Can you work these out from the drawing? Everything is in mm from the part's minimum corner. Give positions to 0.01 mm unless a question says otherwise; leave off trailing zeros. Loops run counter-clockwise (first coordinate to the right, second up) from the corner with the lowest first, then second, coordinate; pieces in that order, holes last.
Q1. If we section it at D-D (z = 20.5): Please give me the cut outline in (x, y), plus the area to 3 significant figures.
Q2. If we section it at A-A (y = 12): Please give me the cut outline in (x, z), plus the area to 4 significant figures.
Q3. Will this pin go through, and if not, where does the flat tip stop? P1, Ø1.5, axis at x = 1.5, z = 18, coming from the -Y side.
Q4. We'd pull the mould along Z, two halves only. Please class the marked faces 1, 2 and 3: +Z half, -Z half, draft (parallel to the pull), parting line (faces both ways), or undercut.
Q5. If we section it at C-C (x = 0.4): Please give me the cut outline in (y, z), plus the area to 3 significant figures.
Q6. I need wall thicknesses on line 1 (Y direction, x = 1.2, z = 12); line 2 (X direction, y = 13.5, z = 21.25). Which ranges of each line are inside material? Lowest first, please.
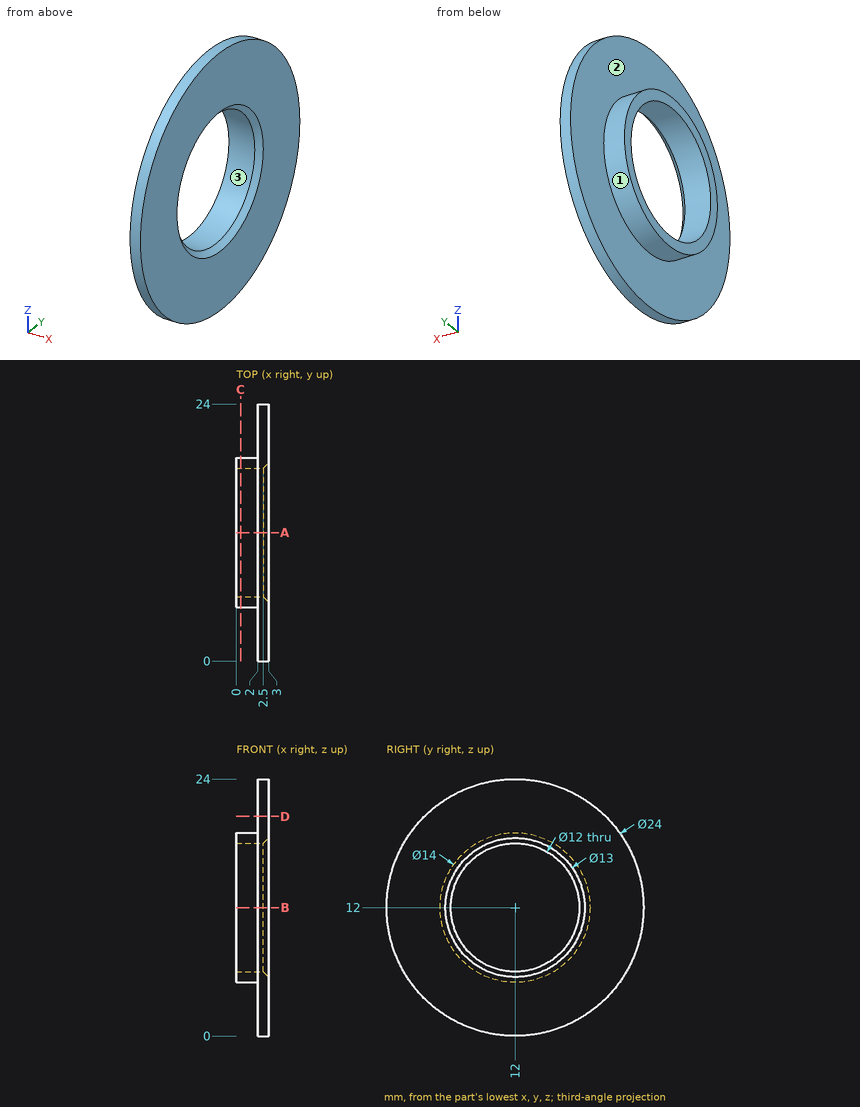
Check sheet entries:
1. outline: (2, 3.53) - (3, 3.53) - (3, 20.47) - (2, 20.47) - close
1. area: 16.9 mm2
2. outline: (0, 5) - (2, 5) - (2, 0) - (3, 0) - (3, 5.5) - (2.5, 6) - (0, 6) - close; (0, 18) - (2.5, 18) - (3, 18.5) - (3, 24) - (2, 24) - (2, 19) - (0, 19) - close
2. area: 15.75 mm2
3. P1: stops at y = 1.3
4. face 1: parting line
4. face 2: draft
4. face 3: undercut
5. outline: circle Ø14 at (12, 12); hole circle Ø12 at (12, 12)
5. area: 40.8 mm2
6. line 1: y = 5 to 6, 18 to 19
6. line 2: x = 2 to 3
